The figure shows three views and two pictorial views of one solid part (mm, origin at its lowest corner). Answer the questions. A direction names the side the tool comes from. Give positions to 0.01 mm unless a question says otherwise; leave off trailing zeros. Loops run counter-clockwise (first coordinate to the right, second up) from the corner with the lowest first, then second, coordinate; pieces in that order, holes last. Notation, with made-up numbers: M 66.25,-19 L 110.25,-19 A29 cw 110.25,19 Z; hole C 7,64 d1. An arc over 180 degrees is marked long. Write item = value, one per line. Start each with the question number.
1. Consider L1, parallel to Y at x = 5.9, z = 1.65; L2, parallel to Y at x = 5, z = 2.3; L3, parallel to X at y = 14.5, z = 1.5. Determine where each line is inside the solid, lowest interval first. Write a range as [from, to].
2. The mould has two halves that part along X. Classify the marked faces 3, 4, 5 and 6: released by +X, released by -X, zero draft, split by the parting line, or undercut.
3. Flat-ended cylindrical pins translate along their axes: pin 1 Ø1.5 at (y, z) = (1.5, 1) entering from -X; pin 2 Ø1.5 at (y, z) = (1.5, 1.5) entering from +X. Find the tip coordinate at first contact, or state that the pin passes through.
4. For the marked faces 1 and 2, determine the directions among +Z, -Z, +X, -X, +Y, -Y from which every point of the face is accessible in a straight line to the end or side of a thin tool.
5. Section C-C on x = 4 is taken. Determine the outline of the cut face in (y, z), plus the area to 3 significant figures.
6. Section B-B on z = 2.1 is taken. Determine the outline of the cut face in (x, y), plus the area to 3 significant figures.
7. Section A-A on y = 8.2 is taken. Determine the outline of the cut face in (x, z).
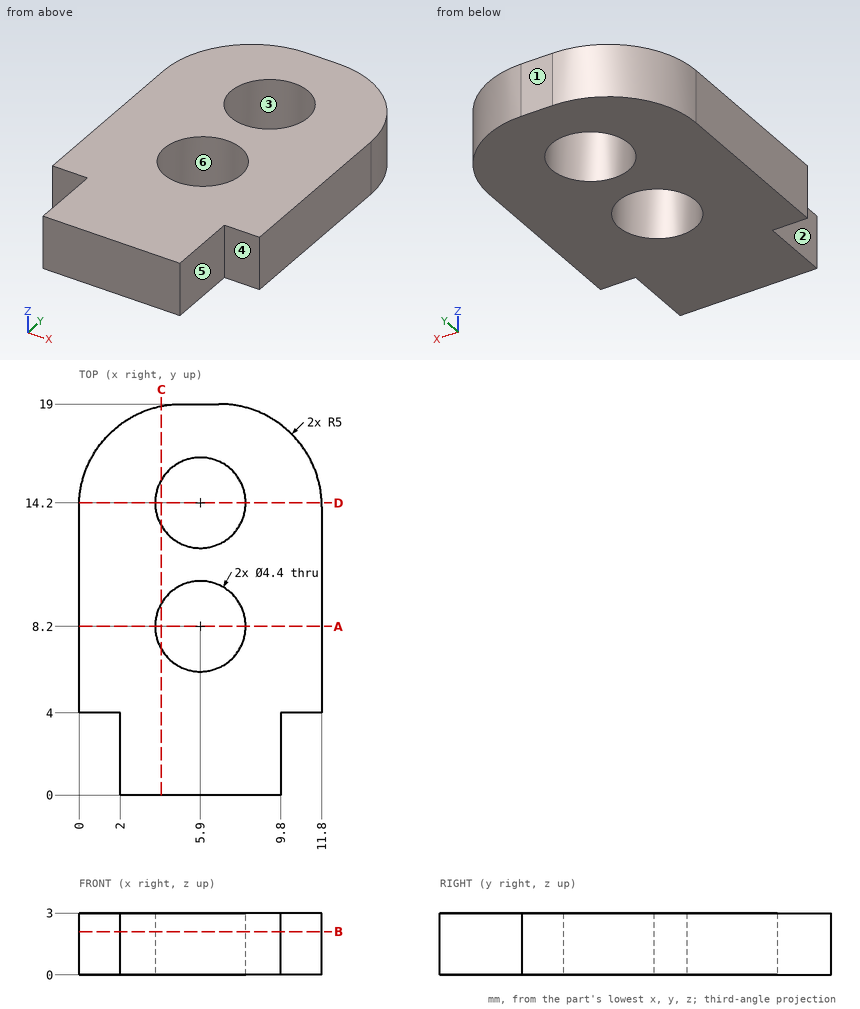
Verdict:
q1.L1 = [0, 6], [10.4, 12], [16.4, 19]
q1.L2 = [0, 6.19], [10.21, 12.19], [16.21, 19]
q1.L3 = [0.03, 3.72], [8.08, 11.77]
q2.face_3 = undercut
q2.face_4 = zero draft
q2.face_5 = released by +X
q2.face_6 = undercut
q3.pin_1 = 2
q3.pin_2 = 9.8
q4.face_1 = +Z, -Z, +X, -X, +Y
q4.face_2 = +Z, -Z, -X, -Y
q5.outline = M 0,0 L 7.09,0 L 7.09,3 L 0,3 Z; M 9.31,0 L 13.09,0 L 13.09,3 L 9.31,3 Z; M 15.31,0 L 18.9,0 L 18.9,3 L 15.31,3 Z
q5.area = 43.4 mm2
q6.outline = M 0,4 L 2,4 L 2,0 L 9.8,0 L 9.8,4 L 11.8,4 L 11.8,14 A5 ccw 6.8,19 L 5,19 A5 ccw 0,14 Z; hole C 5.9,8.2 d4.4; hole C 5.9,14.2 d4.4
q6.area = 167 mm2
q7.outline = M 0,0 L 3.7,0 L 3.7,3 L 0,3 Z; M 8.1,0 L 11.8,0 L 11.8,3 L 8.1,3 Z
